```python
from build123d import *

# Parameters (mm, degrees)
SKETCH1_R               = 3.2639
BOSS_EXTRUDE1_DEPTH     = 6.35
SKETCH6_R               = 3.2639
CUT_EXTRUDE1_DEPTH      = 7.35
CUT_EXTRUDE2_START      = -0.79375
CUT_EXTRUDE2_DEPTH      = 10.82675
CIRPATTERN1_COUNT       = 4
CIRPATTERN1_ANGLE       = 33
BOSS_EXTRUDE2_DEPTH     = 6.35
SKETCH9_R               = 3.2639
CUT_EXTRUDE3_DEPTH      = 1
CUT_EXTRUDE3_DEPTH_BACK = 7.35
FILLET2_R               = 7.9375


with BuildPart() as part:
    # Sketch1 → Boss-Extrude1 (new body)
    with BuildSketch(Plane(origin=(0, 0, 0), x_dir=(0, 0, -1), z_dir=(1, 0, 0))):
        with BuildLine():
            Line((177.8, 0), (177.8, -50.8))
            Line((177.8, -50.8), (228.6, -50.8))
            Line((228.6, -50.8), (228.6, 0))
            ThreePointArc((228.6, 0), (214.813733112, 78.185804764), (175.117759697, 146.941247574))
            Line((175.117759697, 146.941247574), (163.413376386, 153.69877643))
            Line((163.413376386, 153.69877643), (139.091465317, 133.290269822))
            Line((139.091465317, 133.290269822), (136.202701987, 114.287637002))
            ThreePointArc((136.202701987, 114.287637002), (167.077347976, 60.811181483), (177.8, 0))
        make_face()
        with Locations((190.5, -38.1)):
            Circle(SKETCH1_R, mode=Mode.SUBTRACT)
        with Locations((215.9, -38.1)):
            Circle(SKETCH1_R, mode=Mode.SUBTRACT)
    extrude(amount=BOSS_EXTRUDE1_DEPTH)

    # Sketch6 → Cut-Extrude1 (cut, through all)
    with BuildSketch(Plane(origin=(6.35, 0, 0), x_dir=(0, 0, -1), z_dir=(1, 0, 0))):
        with Locations((192.938008153, 16.879888477)):
            Circle(SKETCH6_R)
        with Locations((218.241353484, 19.093644342)):
            Circle(SKETCH6_R)
        with Locations((186.172358961, 53.384064888)):
            Circle(SKETCH6_R)
        with Locations((210.588406038, 60.385253726)):
            Circle(SKETCH6_R)
        with Locations((172.565688572, 87.926610037)):
            Circle(SKETCH6_R)
        with Locations((195.197254287, 99.45796873)):
            Circle(SKETCH6_R)
        with Locations((152.617982705, 119.238236234)):
            Circle(SKETCH6_R)
        with Locations((172.633455846, 134.876037707)):
            Circle(SKETCH6_R)
        with BuildLine():
            Line((192.092529624, 64.990498635), (197.343421252, 46.678463327))
            ThreePointArc((197.343421252, 46.678463327), (202.056006639, 44.066234591), (204.668235375, 48.778819979))
            Line((204.668235375, 48.778819979), (199.417343747, 67.090855286))
            ThreePointArc((199.417343747, 67.090855286), (194.704758359, 69.703084022), (192.092529624, 64.990498635))
        make_face()
        with BuildLine():
            Line((176.162477062, 100.449422723), (184.810996082, 83.475748437))
            ThreePointArc((184.810996082, 83.475748437), (189.935434743, 81.810717384), (191.600465797, 86.935156045))
            Line((191.600465797, 86.935156045), (182.951946777, 103.908830331))
            ThreePointArc((182.951946777, 103.908830331), (177.827508115, 105.573861384), (176.162477062, 100.449422723))
        make_face()
        with BuildLine():
            Line((200.964020569, 27.143457529), (202.624337469, 8.16594853))
            ThreePointArc((202.624337469, 8.16594853), (206.751902648, 4.70251011), (210.215341068, 8.83007529))
            Line((210.215341068, 8.83007529), (208.555024169, 27.807584289))
            ThreePointArc((208.555024169, 27.807584289), (204.427458989, 31.271022709), (200.964020569, 27.143457529))
        make_face()
        with BuildLine():
            Line((159.763864694, 136.908609619), (171.492215799, 121.897004763))
            ThreePointArc((171.492215799, 121.897004763), (170.835565049, 116.549013571), (165.487573857, 117.205664321))
            Line((165.487573857, 117.205664321), (153.759222752, 132.217269177))
            ThreePointArc((153.759222752, 132.217269177), (154.415873502, 137.56526037), (159.763864694, 136.908609619))
        make_face()
    extrude(amount=-CUT_EXTRUDE1_DEPTH, mode=Mode.SUBTRACT)

    # Sketch8 → Cut-Extrude2 (cut)
    with BuildSketch(Plane(origin=(6.35, 15.551634957, -177.756000954), x_dir=(0, 0.087155743, -0.996194698), z_dir=(1, 0, 0)).offset(CUT_EXTRUDE2_START)):
        with BuildLine():
            Line((31.75, 3.175), (24.13, 3.175))
            ThreePointArc((24.13, 3.175), (20.955, 0), (24.13, -3.175))
            Line((24.13, -3.175), (31.75, -3.175))
            ThreePointArc((31.75, -3.175), (34.925, 0), (31.75, 3.175))
        make_face()
    cut_extrude2 = extrude(amount=CUT_EXTRUDE2_DEPTH, mode=Mode.SUBTRACT)

    # CirPattern1: Cut-Extrude2 ×4 about axis
    cirpattern1_axis = Axis((0, 0, 0), (1, 0, 0))
    for i in range(1, CIRPATTERN1_COUNT):
        add(cut_extrude2.rotate(cirpattern1_axis, i * CIRPATTERN1_ANGLE / (CIRPATTERN1_COUNT - 1)), mode=Mode.SUBTRACT)

    # Sketch11 → Boss-Extrude2 (add)
    with BuildSketch(Plane(origin=(6.35, 0, 0), x_dir=(0, 0, -1), z_dir=(1, 0, 0))):
        with BuildLine():
            Line((183.556066953, 163.091467297), (163.413376386, 153.69877643))
            Line((163.413376386, 153.69877643), (175.117759697, 146.941247574))
            ThreePointArc((175.117759697, 146.941247574), (184.855029121, 134.486349525), (193.708175574, 121.388231372))
            Line((193.708175574, 121.388231372), (196.560105656, 153.98594137))
            Line((196.560105656, 153.98594137), (183.556066953, 163.091467297))
        make_face()
    extrude(amount=-BOSS_EXTRUDE2_DEPTH)

    # Sketch9 → Cut-Extrude3 (cut, two sides)
    with BuildSketch(Plane(origin=(6.35, 0, 0), x_dir=(0, 0, -1), z_dir=(1, 0, 0))) as cut_extrude3_sk:
        with Locations((188.512295871, 152.654247257)):
            Circle(SKETCH9_R)
    extrude(amount=CUT_EXTRUDE3_DEPTH, mode=Mode.SUBTRACT)
    extrude(cut_extrude3_sk.sketch, amount=-CUT_EXTRUDE3_DEPTH_BACK, mode=Mode.SUBTRACT)

    # Fillet2
    fillet2_edges = [part.edges().sort_by_distance(p)[0] for p in [
        (3.175, 153.98594137, -196.560105656),
        (3.175, 121.388231372, -193.708175574),
        (3.175, 163.091467297, -183.556066953),
    ]]
    fillet(fillet2_edges, radius=FILLET2_R)


solid = part.part
```
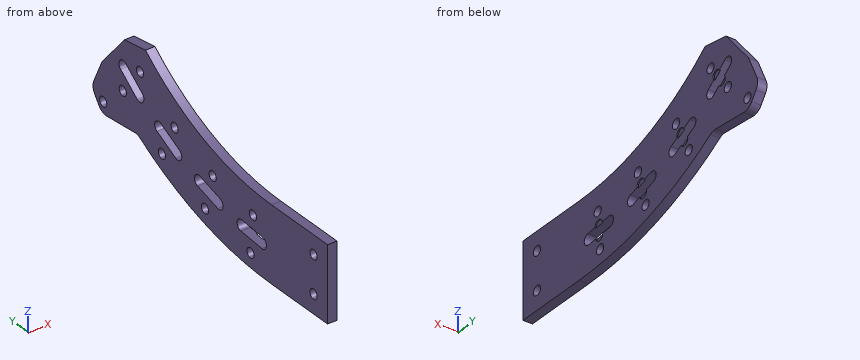
The model under review builds one solid part; all positions refer to its coordinate system, in mm. Coordinates: 2 decimals unless noted, no trailing zeros. Order: outer loops, then holes, each group sorted by start corner. A loop starts at its lowest first (then second) coordinate and runs counter-clockwise, first axis right, second up. Notation, with made-up numbers: (-38.75, 88.5) -> (11.25, 88.5) arc R21 ccw to (11.25, 93.5) -> close; hole circle Ø9 at (41.5, 79). An arc over 180 degrees is marked (long way). Answer in a Markdown table with one row per item. Add a question column.
Item 1: We need section B-B on x = 4.5. Give the number of separate pieces and of enclosed holes in the cut face, plus the area to 3 significant figures.
Item 2: Clearance check with flat-ended pins moving along their axes: pin 1 (6 mm diameter, centred on y = 116, z = -195, fed in from -X); pin 2 (1.5 mm diameter, centred on y = 124.5, z = -159.5, fed in from +X); pin 3 (1.5 mm diameter, centred on x = 2, y = -27.5, fed in from +Z); pin 4 (1.5 mm diameter, centred on x = 1.5, y = 86, fed in from -Z). State where each tip first meets the part, or that it passes through.
Item 3: To check wall thickness, follow probe 1 along Z at (x, y) = (4, -38.5); probe 2 along Z at (x, y) = (6, -39); probe 3 along Z at (x, y) = (3.75, 66). State the ranges of each line that lie inside material, in increasing order.
Item 4: We need section C-C on y = 35. Write out the cut boundary in (x, z), plus the area to 3 significant figures.
Item 5: We need section A-A on y = -38.1. Write out the cut boundary in (x, z).
Final values:
| question | item | result |
|---|---|---|
| 1 | separate pieces | 1 |
| 1 | enclosed holes | 15 |
| 1 | area | 9,770 mm2 |
| 2 | pin 1 | stops at x = 0 |
| 2 | pin 2 | stops at x = 5.56 |
| 2 | pin 3 | stops at z = -177.8 |
| 2 | pin 4 | stops at z = -212.11 |
| 3 | probe 1 | z = -228.6 to -219.14, -212.66 to -193.74, -187.26 to -177.8 |
| 3 | probe 2 | z = -228.6 to -219.04, -212.76 to -193.64, -187.36 to -177.8 |
| 3 | probe 3 | z = -218.87 to -199.73, -191.95 to -165.1 |
| 4 | outline | (0, -225.9) -> (6.35, -225.9) -> (6.35, -174.32) -> (0, -174.32) -> close |
| 4 | area | 328 mm2 |
| 5 | outline | (0, -228.6) -> (6.35, -228.6) -> (6.35, -219.16) -> (0, -219.16) -> close; (0, -212.64) -> (6.35, -212.64) -> (6.35, -193.76) -> (0, -193.76) -> close; (0, -187.24) -> (6.35, -187.24) -> (6.35, -177.8) -> (0, -177.8) -> close |
